Check sheet for the modelled part. Datum: model origin and axes. Units: mm. Round coordinates to 2 decimals unless told otherwise and drop trailing zeros. Write each loop counter-clockwise with the first axis right and the second up, starting at its lowest first coordinate (ties: lowest second). Pieces come first, ordered by that corner, then holes. Notation, with made-up numbers: M -36.5,-18.75 L 9.5,-18.75 A26 cw 9.5,5.25 Z; hole C -14,74 d11. An arc over 180 degrees is marked long. Put each result on its own line as item: value.
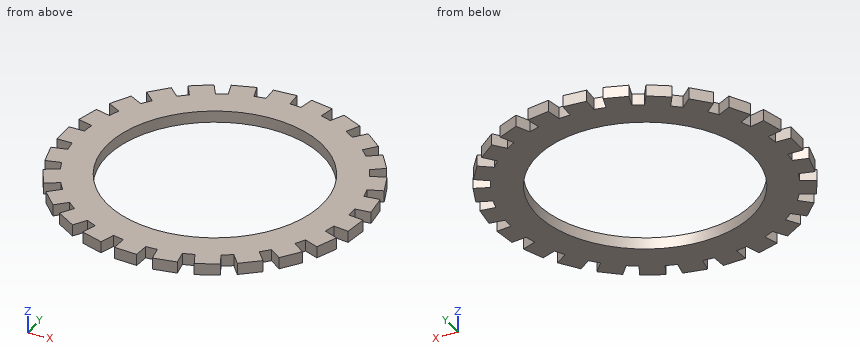
```python
from build123d import *

# Parameters (mm, degrees)
SKETCH1_R           = 226.06
SKETCH1_R_2         = 177.8
BOSS_EXTRUDE1_DEPTH = 19.05
BOSS_EXTRUDE2_START = -19.05
BOSS_EXTRUDE2_DEPTH = 19.05


with BuildPart() as part:
    # Sketch1 → Boss-Extrude1 (new body)
    with BuildSketch(Plane.XY):
        with Locations(Location((0, 0, 0), (0, 0, 180))):
            Circle(SKETCH1_R)
        with Locations(Location((0, 0, 0), (0, 0, 180))):
            Circle(SKETCH1_R_2, mode=Mode.SUBTRACT)
    extrude(amount=BOSS_EXTRUDE1_DEPTH)

    # Sketch2 → Boss-Extrude2 (add)
    with BuildSketch(Plane.XY.offset(19.05).offset(BOSS_EXTRUDE2_START)):
        with BuildLine():
            Line((-250.655901366, 19.05), (-225.255901366, 19.05))
            ThreePointArc((-225.255901366, 19.05), (-226.06, 0), (-225.255901366, -19.05))
            Line((-225.255901366, -19.05), (-250.655901366, -19.05))
            Line((-250.655901366, -19.05), (-250.655901366, 19.05))
        make_face()
        with BuildLine():
            Line((-247.518627651, 43.884078608), (-222.916615358, 37.567355474))
            ThreePointArc((-222.916615358, 37.567355474), (-218.957909405, 56.218835892), (-213.441530657, 74.470373913))
            Line((-213.441530657, 74.470373913), (-238.04354295, 80.787097047))
            Line((-238.04354295, 80.787097047), (-247.518627651, 43.884078608))
        make_face()
        with BuildLine():
            Line((-228.828848251, 104.060759163), (-206.570658578, 91.824215841))
            ThreePointArc((-206.570658578, 91.824215841), (-198.097888091, 108.905235567), (-188.215843594, 125.211500351))
            Line((-188.215843594, 125.211500351), (-210.474033267, 137.448043673))
            Line((-210.474033267, 137.448043673), (-228.828848251, 104.060759163))
        make_face()
        with BuildLine():
            Line((-195.760910741, 157.698919511), (-177.245107605, 140.311423021))
            ThreePointArc((-177.245107605, 140.311423021), (-164.790647915, 154.748718766), (-151.163862869, 168.085127726))
            Line((-151.163862869, 168.085127726), (-169.679666006, 185.472624216))
            Line((-169.679666006, 185.472624216), (-195.760910741, 157.698919511))
        make_face()
        with BuildLine():
            Line((-150.392595252, 201.42827677), (-136.78259466, 179.982347463))
            ThreePointArc((-136.78259466, 179.982347463), (-121.129005273, 190.868770839), (-104.613700698, 200.397348351))
            Line((-104.613700698, 200.397348351), (-118.22370129, 221.843277659))
            Line((-118.22370129, 221.843277659), (-150.392595252, 201.42827677))
        make_face()
        with BuildLine():
            Line((-95.574559898, 232.501154599), (-87.725528241, 208.344319085))
            ThreePointArc((-87.725528241, 208.344319085), (-69.856381748, 214.995836074), (-51.49027497, 220.11786657))
            Line((-51.49027497, 220.11786657), (-59.339306627, 244.274702084))
            Line((-59.339306627, 244.274702084), (-95.574559898, 232.501154599))
        make_face()
        with BuildLine():
            Line((-34.751223446, 248.965129804), (-33.15634425, 223.615250902))
            ThreePointArc((-33.15634425, 223.615250902), (-14.194424845, 225.613922228), (4.868474103, 226.007569696))
            Line((4.868474103, 226.007569696), (3.273594907, 251.357448598))
            Line((3.273594907, 251.357448598), (-34.751223446, 248.965129804))
        make_face()
        with BuildLine():
            Line((28.25566018, 249.785710274), (23.49617479, 224.835614106))
            ThreePointArc((23.49617479, 224.835614106), (42.359419975, 222.0558559), (60.921319042, 217.69638602))
            Line((60.921319042, 217.69638602), (65.680804433, 242.646482188))
            Line((65.680804433, 242.646482188), (28.25566018, 249.785710274))
        make_face()
        with BuildLine():
            Line((89.487136761, 234.91133592), (78.672342755, 211.928728787))
            ThreePointArc((78.672342755, 211.928728787), (96.251666651, 204.54520348), (113.146253454, 195.706537779))
            Line((113.146253454, 195.706537779), (123.96104746, 218.689144911))
            Line((123.96104746, 218.689144911), (89.487136761, 234.91133592))
        make_face()
        with BuildLine():
            Line((145.095807428, 205.276618387), (128.905238088, 185.70558202))
            ThreePointArc((128.905238088, 185.70558202), (144.096067123, 174.182223662), (158.261792638, 161.419728011))
            Line((158.261792638, 161.419728011), (174.452361977, 180.990764377))
            Line((174.452361977, 180.990764377), (145.095807428, 205.276618387))
        make_face()
        with BuildLine():
            Line((191.587574889, 162.743615966), (171.038543232, 147.813870557))
            ThreePointArc((171.038543232, 147.813870557), (182.886381748, 132.874734133), (193.433161344, 116.990323072))
            Line((193.433161344, 116.990323072), (213.982193001, 131.92006848))
            Line((213.982193001, 131.92006848), (191.587574889, 162.743615966))
        make_face()
        with BuildLine():
            Line((226.04119041, 109.984833624), (202.424867669, 100.634469986))
            ThreePointArc((202.424867669, 100.634469986), (210.1852724, 83.21823638), (216.450413126, 65.209985874))
            Line((216.450413126, 65.209985874), (240.066735867, 74.560349512))
            Line((240.066735867, 74.560349512), (226.04119041, 109.984833624))
        make_face()
        with BuildLine():
            Line((246.291806617, 50.31529969), (221.092093203, 47.131835558))
            ThreePointArc((221.092093203, 47.131835558), (224.277449379, 28.33283078), (225.867289402, 9.332265438))
            Line((225.867289402, 9.332265438), (251.067002815, 12.51572957))
            Line((251.067002815, 12.51572957), (246.291806617, 50.31529969))
        make_face()
        with BuildLine():
            Line((251.067002815, -12.51572957), (225.867289402, -9.332265438))
            ThreePointArc((225.867289402, -9.332265438), (224.277449379, -28.33283078), (221.092093203, -47.131835558))
            Line((221.092093203, -47.131835558), (246.291806617, -50.31529969))
            Line((246.291806617, -50.31529969), (251.067002815, -12.51572957))
        make_face()
        with BuildLine():
            Line((240.066735867, -74.560349512), (216.450413126, -65.209985874))
            ThreePointArc((216.450413126, -65.209985874), (210.1852724, -83.21823638), (202.424867669, -100.634469986))
            Line((202.424867669, -100.634469986), (226.04119041, -109.984833624))
            Line((226.04119041, -109.984833624), (240.066735867, -74.560349512))
        make_face()
        with BuildLine():
            Line((213.982193001, -131.92006848), (193.433161344, -116.990323072))
            ThreePointArc((193.433161344, -116.990323072), (182.886381748, -132.874734133), (171.038543232, -147.813870557))
            Line((171.038543232, -147.813870557), (191.587574889, -162.743615966))
            Line((191.587574889, -162.743615966), (213.982193001, -131.92006848))
        make_face()
        with BuildLine():
            Line((174.452361977, -180.990764377), (158.261792638, -161.419728011))
            ThreePointArc((158.261792638, -161.419728011), (144.096067123, -174.182223662), (128.905238088, -185.70558202))
            Line((128.905238088, -185.70558202), (145.095807428, -205.276618387))
            Line((145.095807428, -205.276618387), (174.452361977, -180.990764377))
        make_face()
        with BuildLine():
            Line((123.961047459, -218.689144911), (113.146253454, -195.706537779))
            ThreePointArc((113.146253454, -195.706537779), (96.251666651, -204.54520348), (78.672342755, -211.928728787))
            Line((78.672342755, -211.928728787), (89.487136761, -234.91133592))
            Line((89.487136761, -234.91133592), (123.961047459, -218.689144911))
        make_face()
        with BuildLine():
            Line((65.680804433, -242.646482188), (60.921319042, -217.69638602))
            ThreePointArc((60.921319042, -217.69638602), (42.359419975, -222.0558559), (23.49617479, -224.835614106))
            Line((23.49617479, -224.835614106), (28.25566018, -249.785710274))
            Line((28.25566018, -249.785710274), (65.680804433, -242.646482188))
        make_face()
        with BuildLine():
            Line((3.273594907, -251.357448598), (4.868474103, -226.007569696))
            ThreePointArc((4.868474103, -226.007569696), (-14.194424845, -225.613922228), (-33.15634425, -223.615250902))
            Line((-33.15634425, -223.615250902), (-34.751223446, -248.965129804))
            Line((-34.751223446, -248.965129804), (3.273594907, -251.357448598))
        make_face()
        with BuildLine():
            Line((-59.339306627, -244.274702084), (-51.49027497, -220.11786657))
            ThreePointArc((-51.49027497, -220.11786657), (-69.856381748, -214.995836074), (-87.725528241, -208.344319085))
            Line((-87.725528241, -208.344319085), (-95.574559898, -232.501154599))
            Line((-95.574559898, -232.501154599), (-59.339306627, -244.274702084))
        make_face()
        with BuildLine():
            Line((-118.22370129, -221.843277659), (-104.613700698, -200.397348351))
            ThreePointArc((-104.613700698, -200.397348351), (-121.129005273, -190.868770839), (-136.78259466, -179.982347463))
            Line((-136.78259466, -179.982347463), (-150.392595252, -201.42827677))
            Line((-150.392595252, -201.42827677), (-118.22370129, -221.843277659))
        make_face()
        with BuildLine():
            Line((-169.679666006, -185.472624216), (-151.163862869, -168.085127726))
            ThreePointArc((-151.163862869, -168.085127726), (-164.790647915, -154.748718766), (-177.245107605, -140.311423021))
            Line((-177.245107605, -140.311423021), (-195.760910741, -157.698919511))
            Line((-195.760910741, -157.698919511), (-169.679666006, -185.472624216))
        make_face()
        with BuildLine():
            Line((-210.474033267, -137.448043673), (-188.215843594, -125.211500351))
            ThreePointArc((-188.215843594, -125.211500351), (-198.097888091, -108.905235567), (-206.570658578, -91.824215841))
            Line((-206.570658578, -91.824215841), (-228.828848251, -104.060759163))
            Line((-228.828848251, -104.060759163), (-210.474033267, -137.448043673))
        make_face()
        with BuildLine():
            Line((-238.04354295, -80.787097047), (-213.441530657, -74.470373913))
            ThreePointArc((-213.441530657, -74.470373913), (-218.957909405, -56.218835892), (-222.916615358, -37.567355474))
            Line((-222.916615358, -37.567355474), (-247.518627651, -43.884078608))
            Line((-247.518627651, -43.884078608), (-238.04354295, -80.787097047))
        make_face()
    extrude(amount=BOSS_EXTRUDE2_DEPTH)


solid = part.part
```
1. Cross-section at A-A (y = 0). Enter the section's corners in (x, z), then the cut area to 3 significant figures.
Computed values:
outline: M -250.66,0 L -177.8,0 L -177.8,19.05 L -250.66,19.05 Z; M 177.8,0 L 226.06,0 L 226.06,19.05 L 177.8,19.05 Z
area: 2,310 mm2
2. Depth check by flat-ended pin: pin 1 Ø10 at (y, z) = (-190, 4) entering from +X; pin 2 Ø3 at (y, z) = (-80, 12) entering from -X; pin 3 Ø6 at (y, z) = (-56, 16.5) entering from +X; pin 4 Ø8 at (x, y) = (151.5, -101) entering from -Z. Enter the tip coordinate at first touch or a pass-through.
Computed values:
pin 1: stops at x = 169.61
pin 2: stops at x = -238.63
pin 3: stops at x = 219.76
pin 4: stops at z = 0
3. Cross-section at B-B (x = -43.5). Enter the section's corners in (y, z), then the cut area to 3 significant figures.
Computed values:
outline: M -221.84,0 L -172.4,0 L -172.4,19.05 L -221.84,19.05 Z; M 172.4,0 L 221.84,0 L 221.84,19.05 L 172.4,19.05 Z
area: 1,880 mm2
4. Scan lines: probe 1 along Y at (x, z) = (-207, 8); probe 2 along X at (y, z) = (-153, 5); probe 3 along X at (y, z) = (-162, 10). Record each from-to range of solid material in increasing order.
Computed values:
probe 1: y = -135.54 to -92.06, -90.85 to 90.85, 92.06 to 135.54
probe 2: x = -190.76 to -90.58, 90.58 to 166.42, 178.18 to 198.67
probe 3: x = -191.72 to -73.27, 73.27 to 158.74, 190.56 to 192.13
